```python
from build123d import *

# Parameters (mm, degrees)
BOSS_EXTRUDE1_START     = -12.7
BOSS_EXTRUDE1_DEPTH     = 12.7
F_1_4_CLEARANCE_HOLE1_D = 6.5278
CIRPATTERN1_COUNT       = 3
CHAMFER1_SIZE           = 0.635
CHAMFER1_SIZE2          = 1.744648161


with BuildPart() as part:
    # Sketch1 → Revolve1 (revolve)
    with BuildSketch(Plane.XY, mode=Mode.PRIVATE) as revolve1_sk:
        Polygon((0, 66.675), (23.495, 66.675), (23.495, 63.5), (20.32, 63.5), (20.32, 60.3504), (0, 60.3504), align=None)
    revolve(revolve1_sk.sketch.rotate(Axis((0, 0, 0), (1, 0, 0)), 90), axis=Axis((0, 0, 0), (1, 0, 0)))

    # Sketch5 → Boss-Extrude1 (add)
    with BuildSketch(Plane.ZY.offset(BOSS_EXTRUDE1_START)):
        with BuildLine():
            ThreePointArc((-61.733643772, 45.671707505), (-70.940470951, 40.9575), (-70.41968082, 30.627050022))
            ThreePointArc((-70.41968082, 30.627050022), (-67.700076965, 25.827577718), (-66.080812198, 20.554138506))
            ThreePointArc((-66.080812198, 20.554138506), (-65.542300069, 15.371802621), (-65.894280688, 10.17346537))
            ThreePointArc((-65.894280688, 10.17346537), (-57.742243797, 33.3375), (-41.757619799, 51.979388355))
            ThreePointArc((-41.757619799, 51.979388355), (-46.083521606, 49.075395572), (-50.840812198, 46.950592813))
            ThreePointArc((-50.840812198, 46.950592813), (-56.217376905, 45.716197631), (-61.733643772, 45.671707505))
        make_face()
    boss_extrude1 = extrude(amount=BOSS_EXTRUDE1_DEPTH)

    # 1/4 Clearance Hole1 (through all)
    with Locations(Plane.ZY):
        with Locations((-62.69157898, 36.195)):
            f_1_4_clearance_hole1 = Hole(F_1_4_CLEARANCE_HOLE1_D / 2)

    # CirPattern1: Boss-Extrude1, 1/4 Clearance Hole1 ×3 about axis
    cirpattern1_axis = Axis((0, 0, 0), (1, 0, 0))
    add([boss_extrude1.rotate(cirpattern1_axis, i * 360 / CIRPATTERN1_COUNT) for i in range(1, CIRPATTERN1_COUNT)])
    add([f_1_4_clearance_hole1.rotate(cirpattern1_axis, i * 360 / CIRPATTERN1_COUNT) for i in range(1, CIRPATTERN1_COUNT)], mode=Mode.SUBTRACT)

    # Chamfer1
    chamfer1_edges = [part.edges().sort_by_distance(p)[0] for p in [
        (0, 0, -60.3504),
    ]]
    chamfer1_side = [part.faces().sort_by_distance(p)[0] for p in [
        (0, -36.487585779, 53.312085734),
    ]]
    chamfer(chamfer1_edges, length=CHAMFER1_SIZE, length2=CHAMFER1_SIZE2, reference=chamfer1_side[0])


solid = part.part
```
For this review, take the finished solid that the model builds, in its own axes (mm). A direction names the side the tool comes from. Coordinates: 2 decimals unless noted, no trailing zeros. Order: outer loops, then holes, each group sorted by start corner. A loop starts at its lowest first (then second) coordinate and runs counter-clockwise, first axis right, second up. Notation, with made-up numbers: (-28, -19) - (20, -19) arc R36 cw to (20, 18) - close; hole circle Ø6 at (42.25, 42). An arc over 180 degrees is marked (long way). Answer as a JSON object with one key per item and string values. Group by question number.
1. Clearance check with flat-ended pins moving along their axes: P1, Ø10, axis at y = -69, z = -5, coming from the +X side (3 decimals); P2, Ø6, axis at y = 36.2, z = -62.69, coming from the -X side; P3, Ø7.5, axis at y = 36.2, z = 62.69, coming from the +X side; P4, Ø8, axis at x = 4, z = -40, coming from the -Y side. State where each tip first meets the part, or that it passes through.
2. We need section C-C on x = 6.5. State the section outline as (y, z) points (3 decimals), then the cut area to 3 significant figures.
3. We need section D-D on y = -72.39. State the section outline as (x, z) points, then the cut area to 3 significant figures.
4. For probe 1 along Y at (x, z) = (9.25, 0) (3 decimals); probe 2 along Y at (x, z) = (1.5, -2) (3 decimals); probe 3 along Y at (x, z) = (21, 0) (3 decimals), list the stretches that pass through material, from the lowest coordinate up.
5. We need section B-B on x = 17.25. State the section outline as (y, z) points (3 decimals), then the cut area to 3 significant figures.
6. For faces 1 (the cylindrical face through (21.89, 61.99, -13.77)), 2 (the cylindrical face through (6.44, 25.9, -67.73)), 3 (the cylindrical face through (6.44, 25.76, 67.67)), 4 (the flat face through (12.7, 33, 61)), list the 3-axis set-ups (+Z, -Z, +X, -X, +Y, -Y) from which the entire face can be reached by the end or side of a thin tool; tool diameter is ignored.
7. We need section A-A on y = 0. State the section outline as (x, z) points (3 decimals), then the cut area to 3 significant figures.
8. The part is to be moulded in two halves that separate along Z. For faces 5 (the cylindrical face through (6.439, -71.606, 11.437)), 6 (the cylindrical face through (6.439, 15.445, -65.544)), 7 (the cylindrical face through (6.439, 45.707, 56.294)), say which applies: pulls with the +Z half, pulls with the -Z half, needs draft (parallel to the pull), parting line crosses it, or undercut.
Final values:
{
 "1": {"P1": "x = 23.495", "P2": "through", "P3": "x = 12.7", "P4": "y = -56.12"},
 "2": {"outline": "(-76.299, -8.686) arc R25.4 cw to (-67.505, -15.24) arc R30.48 cw to (-62.153, -24.137) arc R66.675 ccw to (10.173, -65.894) arc R30.48 cw to (20.554, -66.081) arc R25.4 cw to (30.627, -70.42) arc R9.525 ccw to (45.672, -61.734) arc R25.4 cw to (46.951, -50.841) arc R30.48 cw to (51.979, -41.758) arc R66.675 ccw to (51.979, 41.758) arc R30.48 cw to (46.951, 50.841) arc R25.4 cw to (45.672, 61.734) arc R9.525 ccw to (30.627, 70.42) arc R25.4 cw to (20.554, 66.081) arc R30.48 cw to (10.173, 65.894) arc R66.675 ccw to (-62.153, 24.137) arc R30.48 cw to (-67.505, 15.24) arc R25.4 cw to (-76.299, 8.686) arc R9.525 ccw to start; hole circle Ø6.528 at (-72.39, 0); hole circle Ø120.701 at (0, 0); hole circle Ø6.528 at (36.195, -62.692); hole circle Ø6.528 at (36.195, 62.692)", "area": "3,410 mm²"},
 "3": {"outline": "(0, -10.88) - (12.7, -10.88) - (12.7, -3.26) - (0, -3.26) - close; (0, 3.26) - (12.7, 3.26) - (12.7, 10.88) - (0, 10.88) - close", "area": "193 mm²"},
 "4": {"probe 1": "-81.915 to -75.654, -69.126 to -60.35, 60.35 to 66.675", "probe 2": "-81.703 to -74.969, -69.811 to -60.406, 60.406 to 66.645", "probe 3": "-66.675 to -63.5, 63.5 to 66.675"},
 "5": {"outline": "circle Ø133.35 at (0, 0); hole circle Ø120.701 at (0, 0)", "area": "2,520 mm²"},
 "6": {"face 1": "+X", "face 2": "-Z, +X, -X", "face 3": "+Z, +X, -X", "face 4": "+Z, +X, +Y"},
 "7": {"outline": "(0, -66.675) - (23.495, -66.675) - (23.495, -63.5) - (20.32, -63.5) - (20.32, -60.35) - (1.745, -60.35) - (0, -60.985) - close; (0, 60.985) - (1.745, 60.35) - (20.32, 60.35) - (20.32, 63.5) - (23.495, 63.5) - (23.495, 66.675) - (0, 66.675) - close", "area": "276 mm²"},
 "8": {"face 5": "pulls with the +Z half", "face 6": "pulls with the -Z half", "face 7": "undercut"}
}
